Geometry check sheet. Reference: drawing and pictorial views, mm from the part's lowest x, y, z. Round coordinates to 2 decimals unless told otherwise and drop trailing zeros. Write each loop counter-clockwise with the first axis right and the second up, starting at its lowest first coordinate (ties: lowest second). Pieces come first, ordered by that corner, then holes. Notation, with made-up numbers: M -18.5,-33 L 21.5,-33 A31 ccw 21.5,-6 Z; hole C -18.5,66 d11. An arc over 180 degrees is marked long. Answer in a Markdown table with one row per item. Add a question column.
1. Sectioned sample at B-B on z = 1.75. Record the cut outline in (x, y).
2. Go/stop test with flat-tipped pins: pin 1 Ø3 at (x, y) = (56, 86) entering from -Z; pin 2 Ø3.5 at (x, y) = (10, 10) entering from -Z. Record where each tip stops, or that it passes through.
3. Material ranges on probe 1 along Y at (x, z) = (99, 0.8); probe 2 along X at (y, z) = (51.5, 2.05); probe 3 along Y at (x, z) = (65.5, 2.5), recorded low to high.
4. Sectioned sample at A-A on x = 29. Record the cut outline in (y, z).
5. Sectioned sample at C-C on y = 63. Record the cut outline in (x, z).
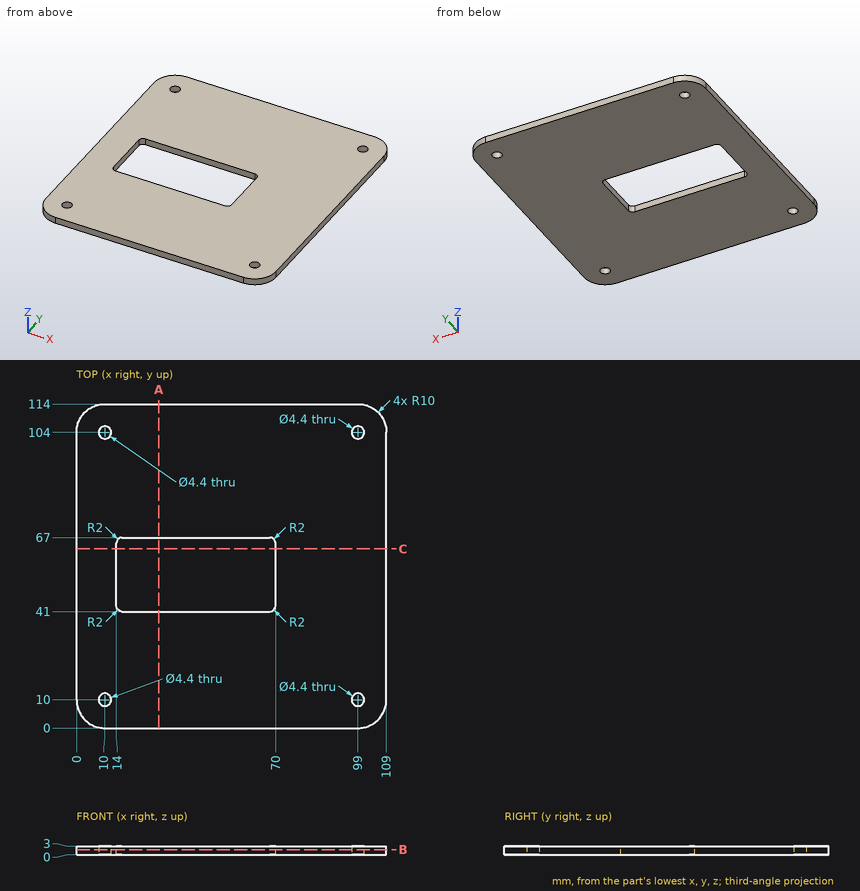
Geometry check:
| question | item | result |
|---|---|---|
| 1 | outline | M 0,10 A10 ccw 10,0 L 99,0 A10 ccw 109,10 L 109,104 A10 ccw 99,114 L 10,114 A10 ccw 0,104 Z; hole C 10,10 d4.4; hole C 10,104 d4.4; hole M 14,43 A2 ccw 16,41 L 68,41 A2 ccw 70,43 L 70,65 A2 ccw 68,67 L 16,67 A2 ccw 14,65 Z; hole C 99,10 d4.4; hole C 99,104 d4.4 |
| 2 | pin 1 | stops at z = 0 |
| 2 | pin 2 | passes through |
| 3 | probe 1 | y = 0 to 7.8, 12.2 to 101.8, 106.2 to 114 |
| 3 | probe 2 | x = 0 to 14, 70 to 109 |
| 3 | probe 3 | y = 0 to 41, 67 to 114 |
| 4 | outline | M 0,0 L 41,0 L 41,3 L 0,3 Z; M 67,0 L 114,0 L 114,3 L 67,3 Z |
| 5 | outline | M 0,0 L 14,0 L 14,3 L 0,3 Z; M 70,0 L 109,0 L 109,3 L 70,3 Z |
